Read the model definition and answer for the solid it produces. Units are mm, in the model's axes. Round coordinates to 2 decimals unless told otherwise and drop trailing zeros. Order: outer loops, then holes, each group sorted by start corner. A loop starts at its lowest first (then second) coordinate and runs counter-clockwise, first axis right, second up. Notation, with made-up numbers: (44, 80) -> (85, 80) arc R11 cw to (85, 95) -> close; hole circle Ø8 at (14, -27). An arc over 180 degrees is marked (long way). Use a Markdown table: item, result. Add a question column.
1. Section D-D, the plane x = 35.5 is taken. Give the vertices of the cut face in (y, z), then the cut area to 3 significant figures.
2. Given pin 1 (9.5 mm diameter, centred on x = 0, y = -32.5, fed in from -Z), flat-ended and moving along its own axis, determine where the tip first touches the part or whether it passes through.
3. Consider L1, parallel to Y at x = 42.5, z = 0.95; L2, parallel to X at y = -40, z = 0.2; L3, parallel to Y at x = -4, z = 0.1. Determine where each line is inside the solid, lowest interval first. Write a range as [from, to].
4. Section A-A, the plane x = -42.5 is taken. Give the vertices of the cut face in (y, z).
5. Section B-B, the plane y = -37 is taken. Give the vertices of the cut face in (x, z).
6. Section C-C, the plane z = 0.4 is taken. Give the number of separate pieces and of enclosed holes in the cut face, then the cut area to 3 significant figures.
```python
from build123d import *

# Parameters (mm, degrees)
ESQUISSE1_W             = 93
ESQUISSE1_H             = 27
ESQUISSE1_R             = 1
BOSS_EXTRU_1_DEPTH      = 1.5
BOSS_EXTRU_2_DEPTH      = 1.5
ESQUISSE3_R             = 6.05
ESQUISSE3_R_2           = 1.5
ENL_V_MAT_EXTRU_1_DEPTH = 69.297144889
CONG_2_R                = 3


with BuildPart() as part:
    # Esquisse1 → Boss.-Extru.1 (new body)
    with BuildSketch(Plane.XY):
        with Locations((0, -13.5)):
            Rectangle(ESQUISSE1_W, ESQUISSE1_H)
        with Locations((42.5, -7)):
            Circle(ESQUISSE1_R, mode=Mode.SUBTRACT)
        with Locations(Location((27.5, -7, 0), (0, 0, 180))):
            Circle(ESQUISSE1_R, mode=Mode.SUBTRACT)
        with Locations(Location((42.5, -20, 0), (0, 0, 180))):
            Circle(ESQUISSE1_R, mode=Mode.SUBTRACT)
        with Locations((27.5, -20)):
            Circle(ESQUISSE1_R, mode=Mode.SUBTRACT)
        with Locations(Location((-42.5, -7, 0), (0, 0, 180))):
            Circle(ESQUISSE1_R, mode=Mode.SUBTRACT)
        with Locations((-42.5, -20)):
            Circle(ESQUISSE1_R, mode=Mode.SUBTRACT)
        with Locations(Location((-27.5, -20, 0), (0, 0, 180))):
            Circle(ESQUISSE1_R, mode=Mode.SUBTRACT)
        with Locations((-27.5, -7)):
            Circle(ESQUISSE1_R, mode=Mode.SUBTRACT)
    extrude(amount=BOSS_EXTRU_1_DEPTH)

    # Esquisse2 → Boss.-Extru.2 (add)
    with BuildSketch(Plane.XY.offset(1.5)):
        with BuildLine():
            Line((-14.428612572, -42.402784419), (-25, -27))
            Line((-25, -27), (25, -27))
            Line((25, -27), (14.428612572, -42.402784419))
            ThreePointArc((14.428612572, -42.402784419), (0, -50), (-14.428612572, -42.402784419))
        make_face()
    extrude(amount=-BOSS_EXTRU_2_DEPTH)

    # Esquisse3 → Enlèv. mat.-Extru.1 (cut, through all)
    with BuildSketch(Plane.XY.offset(1.5)):
        with Locations((0, -32.5)):
            Circle(ESQUISSE3_R)
        with Locations((0, -23.5)):
            Circle(ESQUISSE3_R_2)
        with Locations((5.785088487, -25.605600012)):
            Circle(ESQUISSE3_R_2)
        with Locations((8.863269777, -30.937166401)):
            Circle(ESQUISSE3_R_2)
        with Locations((7.794228634, -37)):
            Circle(ESQUISSE3_R_2)
        with Locations((3.07818129, -40.957233587)):
            Circle(ESQUISSE3_R_2)
        with Locations((-3.07818129, -40.957233587)):
            Circle(ESQUISSE3_R_2)
        with Locations((-7.794228634, -37)):
            Circle(ESQUISSE3_R_2)
        with Locations((-8.863269777, -30.937166401)):
            Circle(ESQUISSE3_R_2)
        with Locations((-5.785088487, -25.605600012)):
            Circle(ESQUISSE3_R_2)
    extrude(amount=-ENL_V_MAT_EXTRU_1_DEPTH, mode=Mode.SUBTRACT)

    # Congé2
    cong_2_edges = [part.edges().sort_by_distance(p)[0] for p in [
        (46.5, 0, 0.75),
        (46.5, -27, 0.75),
        (-46.5, -27, 0.75),
        (-46.5, 0, 0.75),
        (25, -27, 0.75),
        (-25, -27, 0.75),
    ]]
    fillet(cong_2_edges, radius=CONG_2_R)


solid = part.part
```
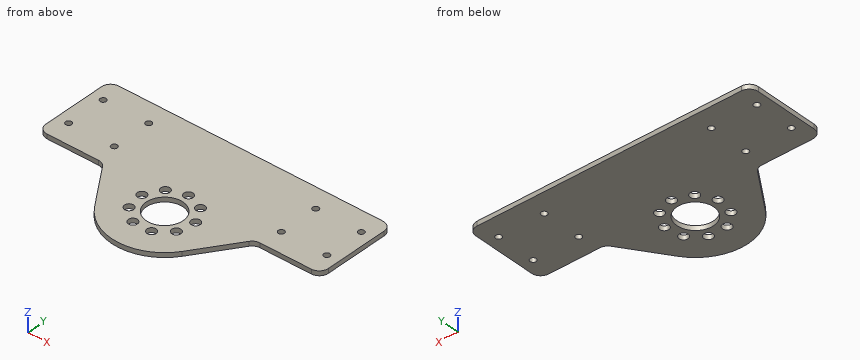
Verdict:
| question | item | result |
|---|---|---|
| 1 | outline | (-27, 0) -> (0, 0) -> (0, 1.5) -> (-27, 1.5) -> close |
| 1 | area | 40.5 mm2 |
| 2 | pin 1 | passes through |
| 3 | L1 | y = [-27, -21], [-19, -8], [-6, 0] |
| 3 | L2 | x = [-16.08, -4.23], [-1.92, 1.92], [4.23, 16.08] |
| 3 | L3 | y = [-49.54, -42.14], [-39.77, -37.04], [-27.96, 0] |
| 4 | outline | (-27, 0) -> (-21, 0) -> (-21, 1.5) -> (-27, 1.5) -> close; (-19, 0) -> (-8, 0) -> (-8, 1.5) -> (-19, 1.5) -> close; (-6, 0) -> (0, 0) -> (0, 1.5) -> (-6, 1.5) -> close |
| 5 | outline | (-18.14, 0) -> (-9.29, 0) -> (-9.29, 1.5) -> (-18.14, 1.5) -> close; (-6.29, 0) -> (-4.04, 0) -> (-4.04, 1.5) -> (-6.29, 1.5) -> close; (4.04, 0) -> (6.29, 0) -> (6.29, 1.5) -> (4.04, 1.5) -> close; (9.29, 0) -> (18.14, 0) -> (18.14, 1.5) -> (9.29, 1.5) -> close |
| 6 | separate pieces | 1 |
| 6 | enclosed holes | 18 |
| 6 | area | 3,060 mm2 |
